```python
from build123d import *

# Parameters (mm, degrees)
EXTRUDE_1_DEPTH     = 5
SKETCH_2_R          = 28
SKETCH_2_R_2        = 26
EXTRUDE_2_DEPTH     = 16
SKETCH_3_R          = 1.65
CUT_EXTRUDE_1_DEPTH = 91.573676352
CHAMFER_1_SIZE      = 3
CHAMFER_1_SIZE_2    = 13


with BuildPart() as part:
    # 草图1 → 凸台-拉伸1 (new body)
    with BuildSketch(Plane.XY):
        with BuildLine():
            Line((-23.815698604, 51.25), (-56.291651246, -5))
            ThreePointArc((-56.291651246, -5), (-56.291651246, -32.5), (-32.475952642, -46.25))
            Line((-32.475952642, -46.25), (32.475952642, -46.25))
            ThreePointArc((32.475952642, -46.25), (56.291651246, -32.5), (56.291651246, -5))
            Line((56.291651246, -5), (23.815698604, 51.25))
            ThreePointArc((23.815698604, 51.25), (0, 65), (-23.815698604, 51.25))
        make_face()
    extrude(amount=EXTRUDE_1_DEPTH)

    # 草图2 → 凸台-拉伸2 (add)
    # profile 1 of 3: a face of its own
    with BuildSketch(Plane.XY.offset(5)):
        with Locations(Location((0, 37.5, 0), (0, 0, 160.844062564))):
            Circle(SKETCH_2_R)
        with Locations((0, 37.5)):
            Circle(SKETCH_2_R_2, mode=Mode.SUBTRACT)
    # profile 2 of 3: a face of its own
    with BuildSketch(Plane.XY.offset(5)):
        with Locations(Location((32.475952642, -18.75, 0), (0, 0, 259.155937436))):
            Circle(SKETCH_2_R)
        with Locations((32.475952642, -18.75)):
            Circle(SKETCH_2_R_2, mode=Mode.SUBTRACT)
    # profile 3 of 3: a face of its own
    with BuildSketch(Plane.XY.offset(5)):
        with Locations(Location((-32.475952642, -18.75, 0), (0, 0, 139.155937436))):
            Circle(SKETCH_2_R)
        with Locations((-32.475952642, -18.75)):
            Circle(SKETCH_2_R_2, mode=Mode.SUBTRACT)
    extrude(amount=EXTRUDE_2_DEPTH)

    # 草图3 → 切除-拉伸1 (cut, through all)
    with BuildSketch(Plane.XY.offset(5)):
        Circle(SKETCH_3_R)
        with Locations((-1.811733316, 6.761480784)):
            Circle(SKETCH_3_R)
        with Locations((6.761480784, 1.811733316)):
            Circle(SKETCH_3_R)
        with Locations((1.811733316, -6.761480784)):
            Circle(SKETCH_3_R)
        with Locations((-6.761480784, -1.811733316)):
            Circle(SKETCH_3_R)
    extrude(amount=-CUT_EXTRUDE_1_DEPTH, mode=Mode.SUBTRACT)

    # 倒角1
    # the kernel refuses this chamfer: 13, 3 mm, written as the material it takes off along each edge
    with BuildSketch(Plane(origin=(-32.475952642, -18.75, 21), x_dir=(1, 0, 0), z_dir=(0, -1, 0))) as chamfer_1_piece_1:
        Polygon((26 + CHAMFER_1_SIZE, 0), (26, -CHAMFER_1_SIZE_2), (26, 0), align=None)
    revolve(axis=Axis((-32.475952642, -18.75, 21), (0, 0, 1)), mode=Mode.SUBTRACT)
    with BuildSketch(Plane(origin=(32.475952642, -18.75, 21), x_dir=(1, 0, 0), z_dir=(0, -1, 0))) as chamfer_1_piece_2:
        Polygon((26 + CHAMFER_1_SIZE, 0), (26, -CHAMFER_1_SIZE_2), (26, 0), align=None)
    revolve(axis=Axis((32.475952642, -18.75, 21), (0, 0, 1)), mode=Mode.SUBTRACT)
    with BuildSketch(Plane(origin=(0, 37.5, 21), x_dir=(1, 0, 0), z_dir=(0, -1, 0))) as chamfer_1_piece_3:
        Polygon((26 + CHAMFER_1_SIZE, 0), (26, -CHAMFER_1_SIZE_2), (26, 0), align=None)
    revolve(axis=Axis((0, 37.5, 21), (0, 0, 1)), mode=Mode.SUBTRACT)


solid = part.part
```
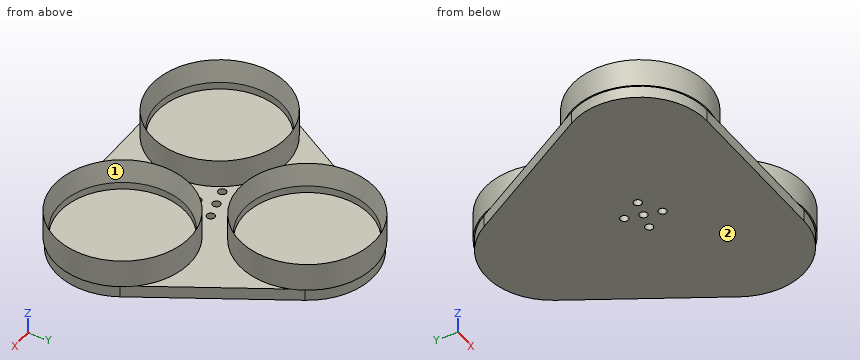
Geometry check sheet. Reference: the model listing, model coordinates, mm. Face numbers are marked on the shaded views. Coordinates: 2 decimals unless noted, no trailing zeros. Write each loop counter-clockwise with the first axis right and the second up, starting at its lowest first coordinate (ties: lowest second). Pieces come first, ordered by that corner, then holes. Notation, with made-up numbers: (42.25, 65) -> (92.25, 65) arc R13 cw to (92.25, 74) -> close; hole circle Ø5 at (-10.5, 65.25). An arc over 180 degrees is marked (long way). Use CSV: the item, a comma, the result in double quotes. Start each with the question number.
Item 1: Cross-section at B-B, the plane y = -18.75. Record the cut outline in (x, z).
Item 2: Thickness scan on line 1 (X direction, y = -22, z = 10.75); line 2 (Y direction, x = 12, z = 15); line 3 (Y direction, x = 0, z = 1.7). Record the ranges inside material, lowest first.
Item 3: Depth check by flat-ended pin: pin 1 Ø4 at (x, z) = (1, 3.5) entering from -Y; pin 2 Ø10 at (y, z) = (40, 11) entering from +X; pin 3 Ø2 at (y, z) = (19.5, 12) entering from -X. Enter the tip coordinate at first touch or a pass-through.
Item 4: Cross-section at A-A, the plane z = 13.25. Record the cut outline in (x, y).
Item 5: Cross-section at C-C, the plane y = 37.5. Record the cut outline in (x, z), plus the area to 3 significant figures.
Item 6: Mould release check, pull along Y, two halves, no side actions. Record for the marked faces 1 and 2: released by +Y, released by -Y, zero draft, split by the parting line, or undercut.
Answers:
1,outline,"(-60.48, 5) -> (-59.98, 5) -> (-59.98, 0) -> (59.98, 0) -> (59.98, 5) -> (60.48, 5) -> (60.48, 16.67) -> (58.48, 8) -> (58.48, 5) -> (6.48, 5) -> (6.48, 8) -> (4.48, 16.67) -> (4.48, 5) -> (-4.48, 5) -> (-4.48, 16.67) -> (-6.48, 8) -> (-6.48, 5) -> (-58.48, 5) -> (-58.48, 8) -> (-60.48, 16.67) -> close"
2,line 1,"-60.29 to -58.91, -6.04 to -4.67, 4.67 to 6.04, 58.91 to 60.29"
2,line 2,"-37.85 to -37.28, -0.22 to 0.35, 12.2 to 12.63, 62.37 to 62.8"
2,line 3,"-46.25 to -1.65, 1.65 to 65"
3,pin 1,"y = -46.25"
3,pin 2,"x = 28"
3,pin 3,"x = -22.25"
4,outline,"circle Ø56 at (-32.48, -18.75); circle Ø56 at (0, 37.5); circle Ø56 at (32.48, -18.75); hole circle Ø54.42 at (-32.48, -18.75); hole circle Ø54.42 at (0, 37.5); hole circle Ø54.42 at (32.48, -18.75)"
5,outline,"(-31.75, 0) -> (31.75, 0) -> (31.75, 5) -> (28, 5) -> (28, 16.67) -> (26, 8) -> (26, 5) -> (-26, 5) -> (-26, 8) -> (-28, 16.67) -> (-28, 5) -> (-31.75, 5) -> close"
5,area,"347 mm^2"
6,face 1,"undercut"
6,face 2,"zero draft"
